The listing builds one solid part. Answer for the finished solid, in the listing's coordinates (mm). Round coordinates to 2 decimals unless told otherwise and drop trailing zeros. Write each loop counter-clockwise with the first axis right and the second up, starting at its lowest first coordinate (ties: lowest second). Pieces come first, ordered by that corner, then holes. Notation, with made-up numbers: (70, 42) - (91, 42) arc R3 cw to (91, 46) - close; hole circle Ø5 at (23.25, -37.5). An arc over 180 degrees is marked (long way). Return JSON: item names as keys, results as strings. Group by question number.
(1) Section A-A, the plane x = 85 is taken. Write down the section's boundary in (y, z), then the cut area to 3 significant figures.
(2) Section B-B, the plane y = 2.45 is taken. Write down the section's boundary in (x, z), then the cut area to 3 significant figures.
(3) Find the intervals of material crossed by line 1 along X through (y, z) = (4.5, 0); line 2 along Z through (x, y) = (85, 2.1); line 3 along X through (y, z) = (0.7, -9), in increasing order. Write a range as [from, to].
(4) This flat-tipped pin is pushed along its axis until it touches: pin 1 (3.5 mm diameter, centred on x = -85, z = 0, fed in from +Y). Where does it stop, or does it pass through?
(5) Section C-C, the plane z = 0 is taken. Write down the section's boundary in (x, y).
(6) Section D-D, the plane x = -85 is taken. Write down the section's boundary in (y, z).
```python
from build123d import *

# Parameters (mm, degrees)
SKETCH2_R           = 5
SKETCH2_R_2         = 3
SKETCH2_W           = 6
SKETCH2_H           = 25
BOSS_EXTRUDE1_DEPTH = 6


with BuildPart() as part:
    # Sketch2 → Boss-Extrude1 (new body)
    with BuildSketch(Plane(origin=(0, 0, 0), x_dir=(1, 0, 0), z_dir=(0, 1, 0))):
        with BuildLine():
            Line((-90, 20), (90, 20))
            ThreePointArc((90, 20), (97.071067812, 17.071067812), (100, 10))
            Line((100, 10), (100, -10))
            ThreePointArc((100, -10), (97.071067812, -17.071067812), (90, -20))
            Line((90, -20), (-90, -20))
            ThreePointArc((-90, -20), (-97.071067812, -17.071067812), (-100, -10))
            Line((-100, -10), (-100, 10))
            ThreePointArc((-100, 10), (-97.071067812, 17.071067812), (-90, 20))
        make_face()
        with Locations((85, 0)):
            Circle(SKETCH2_R, mode=Mode.SUBTRACT)
        with Locations((-85, 0)):
            Circle(SKETCH2_R_2, mode=Mode.SUBTRACT)
        with Locations((-36, 0)):
            Rectangle(SKETCH2_W, SKETCH2_H, mode=Mode.SUBTRACT)
    extrude(amount=BOSS_EXTRUDE1_DEPTH)


solid = part.part
```
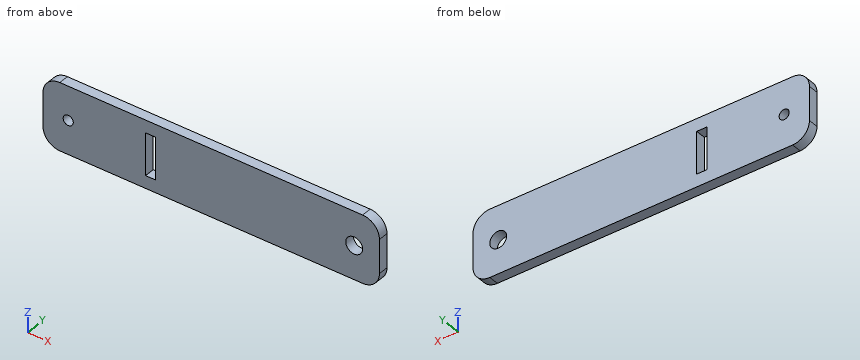
Working result:
{
 "1": {"outline": "(0, -20) - (6, -20) - (6, -5) - (0, -5) - close; (0, 5) - (6, 5) - (6, 20) - (0, 20) - close", "area": "180 mm^2"},
 "2": {"outline": "(-100, -10) arc R10 ccw to (-90, -20) - (90, -20) arc R10 ccw to (100, -10) - (100, 10) arc R10 ccw to (90, 20) - (-90, 20) arc R10 ccw to (-100, 10) - close; hole circle Ø6 at (-85, 0); hole (-39, -12.5) - (-33, -12.5) - (-33, 12.5) - (-39, 12.5) - close; hole circle Ø10 at (85, 0)", "area": "7,660 mm^2"},
 "3": {"line 1": "x = [-100, -88], [-82, -39], [-33, 80], [90, 100]", "line 2": "z = [-20, -5], [5, 20]", "line 3": "x = [-100, -39], [-33, 100]"},
 "4": {"pin 1": "passes through"},
 "5": {"outline": "(-100, 0) - (-88, 0) - (-88, 6) - (-100, 6) - close; (-82, 0) - (-39, 0) - (-39, 6) - (-82, 6) - close; (-33, 0) - (80, 0) - (80, 6) - (-33, 6) - close; (90, 0) - (100, 0) - (100, 6) - (90, 6) - close"},
 "6": {"outline": "(0, -20) - (6, -20) - (6, -3) - (0, -3) - close; (0, 3) - (6, 3) - (6, 20) - (0, 20) - close"}
}
